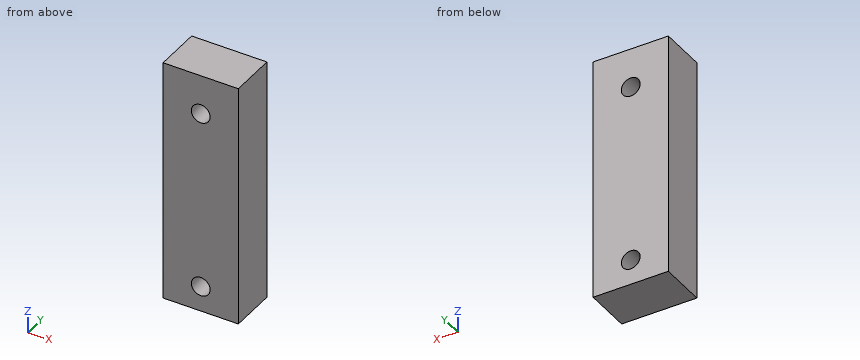
Autodesk Inventor part; units mm, degrees
ref_plane "YZ Plane" through (0, 0, 0) normal (1, 0, 0) x (0, 1, 0)
ref_plane "XZ Plane" through (0, 0, 0) normal (0, 1, 0) x (-1, 0, 0)
ref_plane "XY Plane" through (0, 0, 0) normal (0, 0, 1) x (1, 0, 0)
sketch "Sketch1" plane through (0, 0, 0) normal (0, 0, 1) x (1, 0, 0)
  line L0 (-4, 2.5) -> (4, 2.5)
  line L1 (4, 2.5) -> (4, -2.5)
  line L2 (4, -2.5) -> (-4, -2.5)
  line L3 (-4, -2.5) -> (-4, 2.5)
  line L4 (-4, 2.5) -> (4, -2.5) construction
  line L5 (4, 2.5) -> (-4, -2.5) construction
  point P0 (0, 0)
  dimension "d0" = 8
  dimension "d1" = 5
extrude "Extrusion1" add sketch "Sketch1" along normal blind 25
sketch "Sketch2" plane through (-4, -2.5, 0) normal (0, -1, 0) x (1, 0, 0)
  circle A0 centre (4, 1.7) radius 1
  circle A1 centre (4, 20.8) radius 1
  point P0 (4, 0)
  dimension "d4" = 2
  dimension "d5" = 2
extrude "Extrusion2" cut sketch "Sketch2" against normal up to next
sketch "Sketch3" plane through (0, 0, 0) normal (0, 0, -1) x (-1, 0, 0)
  line L0 (-4, -2.5) -> (4, -2.5)
  line L1 (-4, -2.5) -> (-4, 2.5)
  line L2 (4, -2.5) -> (-4, -2.5)
  line L3 (-4, -2.5) -> (-4, 2.5)
  line L4 (-4, 2.5) -> (4, 2.5)
  line L5 (4, 2.5) -> (4, -2.5)
  point P0 (0, 0)
extrude "Extrusion3" add sketch "Sketch3" along normal blind 1
properties part number "支架 assembly"
Source: CAD feature listing. Evaluate the final solid. Frame: model axes, mm. Coordinates: 2 decimals unless noted, no trailing zeros. Write each loop counter-clockwise with the first axis right and the second up, starting at its lowest first coordinate (ties: lowest second). Pieces come first, ordered by that corner, then holes. Notation, with made-up numbers: (13, 7.25) -> (25, 7.25) arc R22 cw to (25, 30.25) -> close; hole circle Ø1 at (77, 32.25). An arc over 180 degrees is marked (long way). Return JSON: item names as keys, results as strings. Group by question number.
1) Section query D-D, the plane z = 1. Return loops of the section in (x, y).
2) Contact query for a flat-ended pin moving along its axis: P1, Ø1.2, axis at x = 0, z = 1.7, coming from the -Y side. Output: stop coordinate, or through.
3) Section query B-B, the plane x = 0. Return loops of the section in (y, z), plus the area to 3 significant figures.
4) Section query A-A, the plane z = 20.8. Return loops of the section in (x, y), plus the area to 3 significant figures.
5) Section query C-C, the plane y = -0.65. Return loops of the section in (x, z), plus the area to 3 significant figures.
6) Ray query, line 1 along Z through (x, y) = (0, -0.8); line 2 along X through (y, z) = (0.9, 20). Return the intervals inside material, ascending.
From the geometry:
{
 "1": {"outline": "(-4, -2.5) -> (-0.71, -2.5) -> (-0.71, 2.5) -> (-4, 2.5) -> close; (0.71, -2.5) -> (4, -2.5) -> (4, 2.5) -> (0.71, 2.5) -> close"},
 "2": {"P1": "through"},
 "3": {"outline": "(-2.5, -1) -> (2.5, -1) -> (2.5, 0.7) -> (-2.5, 0.7) -> close; (-2.5, 2.7) -> (2.5, 2.7) -> (2.5, 19.8) -> (-2.5, 19.8) -> close; (-2.5, 21.8) -> (2.5, 21.8) -> (2.5, 25) -> (-2.5, 25) -> close", "area": "110 mm²"},
 "4": {"outline": "(-4, -2.5) -> (-1, -2.5) -> (-1, 2.5) -> (-4, 2.5) -> close; (1, -2.5) -> (4, -2.5) -> (4, 2.5) -> (1, 2.5) -> close", "area": "30.0 mm²"},
 "5": {"outline": "(-4, -1) -> (4, -1) -> (4, 25) -> (-4, 25) -> close; hole circle Ø2 at (0, 1.7); hole circle Ø2 at (0, 20.8)", "area": "202 mm²"},
 "6": {"line 1": "-1 to 0.7, 2.7 to 19.8, 21.8 to 25", "line 2": "-4 to -0.6, 0.6 to 4"}
}
